Read the model definition and answer for the solid it produces. Units are mm, in the model's axes. A direction names the side the tool comes from. Give positions to 0.01 mm unless a question says otherwise; leave off trailing zeros. Write each loop counter-clockwise with the first axis right and the second up, starting at its lowest first coordinate (ties: lowest second). Pieces come first, ordered by that corner, then holes. Notation, with made-up numbers: (79.5, 70) -> (101.5, 70) arc R21 cw to (101.5, 79) -> close; hole circle Ø3 at (20, 52.5). An arc over 180 degrees is marked (long way). Use a Markdown table: item, result.
from build123d import *

# Parameters (mm, degrees)
EXTRUDE_1_DEPTH     = 14
SKETCH_2_R          = 2.75
CUT_EXTRUDE_1_DEPTH = 14
FILLET_1_R          = 1


with BuildPart() as part:
    # 草图1 → 凸台-拉伸1 (new body)
    with BuildSketch(Plane.XY):
        with BuildLine():
            Line((-0.5, 33), (-8, 33))
            ThreePointArc((-8, 33), (-8.707106781, 32.707106781), (-9, 32))
            Line((-9, 32), (-9, 7.5))
            ThreePointArc((-9, 7.5), (-9.292893219, 6.792893219), (-10, 6.5))
            Line((-10, 6.5), (-19.9, 6.5))
            ThreePointArc((-19.9, 6.5), (-20.607106781, 6.207106781), (-20.9, 5.5))
            Line((-20.9, 5.5), (-20.9, 1))
            ThreePointArc((-20.9, 1), (-20.607106781, 0.292893219), (-19.9, 0))
            Line((-19.9, 0), (19.9, 0))
            ThreePointArc((19.9, 0), (20.607106781, 0.292893219), (20.9, 1))
            Line((20.9, 1), (20.9, 5.5))
            ThreePointArc((20.9, 5.5), (20.607106781, 6.207106781), (19.9, 6.5))
            Line((19.9, 6.5), (10, 6.5))
            ThreePointArc((10, 6.5), (9.292893219, 6.792893219), (9, 7.5))
            Line((9, 7.5), (9, 32))
            ThreePointArc((9, 32), (8.707106781, 32.707106781), (8, 33))
            Line((8, 33), (0.5, 33))
            Line((0.5, 33), (0.5, 23.468626967))
            ThreePointArc((0.5, 23.468626967), (0, 15.5), (-0.5, 23.468626967))
            Line((-0.5, 23.468626967), (-0.5, 33))
        make_face()
    extrude(amount=EXTRUDE_1_DEPTH)

    # 草图2 → 切除-拉伸1 (cut)
    with BuildSketch(Plane(origin=(0, 0, 0), x_dir=(1, 0, 0), z_dir=(0, 1, 0))):
        with Locations((16.15, -7)):
            Circle(SKETCH_2_R)
        with Locations(Location((-16.15, -7, 0), (0, 0, 90))):
            Circle(SKETCH_2_R)
    extrude(amount=CUT_EXTRUDE_1_DEPTH, mode=Mode.SUBTRACT)

    # 圆角1
    fillet_1_edges = [part.edges().sort_by_distance(p)[0] for p in [
        (13.4, 0, 7),
        (13.4, 6.5, 7),
        (-16.15, 0, 9.75),
        (-16.15, 6.5, 9.75),
    ]]
    fillet(fillet_1_edges, radius=FILLET_1_R - 0.0001)  # a hair under: the kernel refuses the full size


solid = part.part
Item 1: A cutting plane is placed at B-B (y = 19.5). Give the vertices of the cut face in (x, z).
Return value:
| item | result |
|---|---|
| outline | (-9, 0) -> (-4, 0) -> (-4, 14) -> (-9, 14) -> close; (4, 0) -> (9, 0) -> (9, 14) -> (4, 14) -> close |
Item 2: Straight lines are drawn through the part: line 1 along X through (y, z) = (3.2, 7); line 2 along X through (y, z) = (30.5, 10.5); line 3 along Z through (x, y) = (16, 2). For each, find the intervals that lie inside material, in ascending order. Write a range as [from, to].
Return value:
| item | result |
|---|---|
| line 1 | [-20.9, -18.9], [-13.4, 13.4], [18.9, 20.9] |
| line 2 | [-9, -0.5], [0.5, 9] |
| line 3 | [0, 4.25], [9.75, 14] |
Item 3: A cutting plane is placed at A-A (x = 16.15). Give the vertices of the cut face in (y, z).
Return value:
| item | result |
|---|---|
| outline | (0, 0) -> (6.5, 0) -> (6.5, 3.25) arc R1 ccw to (5.5, 4.25) -> (1, 4.25) arc R1 ccw to (0, 3.25) -> close; (0, 10.75) arc R1 ccw to (1, 9.75) -> (5.5, 9.75) arc R1 ccw to (6.5, 10.75) -> (6.5, 14) -> (0, 14) -> close |
Item 4: Each of these flat-tipped pins is pushed along its axis until it touches: P1, Ø8, axis at x = 15.5, z = 9.5, coming from the +Y side; P2, Ø5, axis at y = 9.5, z = 10, coming from the -X side. Where does it stop, or does it pass through?
Return value:
| item | result |
|---|---|
| P1 | y = 6.5 |
| P2 | x = -9.13 |
Item 5: For a pull along Z with two mould halves and no side action, classify faces 1 (the face through (-18.877, 3.218, 7.358)), 2 (the face through (20.599, 0.285, 6.902)), 3 (the face through (0, 13, 14)) as +Z half, -Z half, draft (parallel to the pull), parting line (faces both ways), or undercut.
Return value:
| item | result |
|---|---|
| face 1 | undercut |
| face 2 | draft |
| face 3 | +Z half |
Item 6: A cutting plane is placed at C-C (y = 2). Give the vertices of the cut face in (x, z), then the cut area to 3 significant figures.
Return value:
| item | result |
|---|---|
| outline | (-20.9, 0) -> (20.9, 0) -> (20.9, 14) -> (-20.9, 14) -> close; hole circle Ø5.5 at (-16.15, 7); hole circle Ø5.5 at (16.15, 7) |
| area | 538 mm^2 |
Item 7: A tool of negligible diameter and unlimited length cuts with its end or side. For faces 4 (the face through (0, 0, 7)), 5 (the face through (-4, 33, 7)), 6 (the face through (9, 20, 7)), 7 (the face through (-0.5, 28, 7)), 8 (the face through (-9, 20, 7)), from which of +Z, -Z, +X, -X, +Y, -Y can it reach the whole face along a straight path? Write none if from no direction.
Return value:
| item | result |
|---|---|
| face 4 | +Z, -Z, +X, -X, -Y |
| face 5 | +Z, -Z, +X, -X, +Y |
| face 6 | +Z, -Z, +X, +Y |
| face 7 | +Z, -Z, +Y |
| face 8 | +Z, -Z, -X, +Y |
Item 8: A cutting plane is placed at D-D (z = 2). Give the vertices of the cut face in (x, y), then the cut area to 3 significant figures.
Return value:
| item | result |
|---|---|
| outline | (-20.9, 1) arc R1 ccw to (-19.9, 0) -> (19.9, 0) arc R1 ccw to (20.9, 1) -> (20.9, 5.5) arc R1 ccw to (19.9, 6.5) -> (10, 6.5) arc R1 cw to (9, 7.5) -> (9, 32) arc R1 ccw to (8, 33) -> (0.5, 33) -> (0.5, 23.47) arc R4 cw (long way) to (-0.5, 23.47) -> (-0.5, 33) -> (-8, 33) arc R1 ccw to (-9, 32) -> (-9, 7.5) arc R1 cw to (-10, 6.5) -> (-19.9, 6.5) arc R1 ccw to (-20.9, 5.5) -> close |
| area | 688 mm^2 |
